Check sheet for the modelled part. Datum: model origin and axes. Units: mm. Face numbers are marked on the shaded views. A direction names the side the tool comes from. Coordinates: 2 decimals unless noted, no trailing zeros. Loops run counter-clockwise (first coordinate to the right, second up) from the corner with the lowest first, then second, coordinate; pieces in that order, holes last. Notation, with made-up numbers: (14.5, 32.25) -> (26.5, 32.25) arc R24 ccw to (26.5, 42.25) -> close; hole circle Ø3 at (-3, -17.5). An arc over 180 degrees is marked (long way). Use CSV: the item, a comma, the result in double quotes.
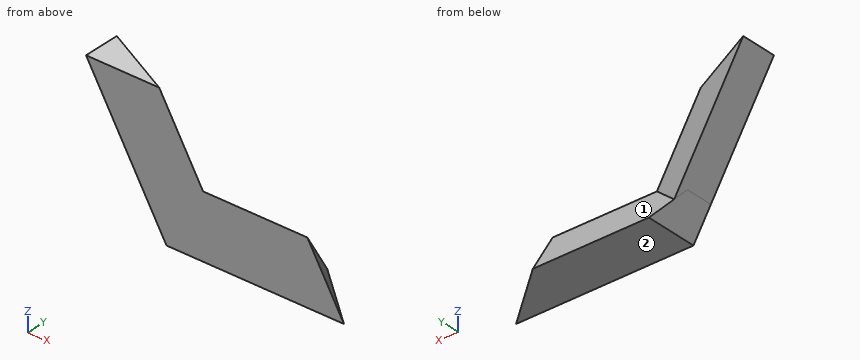
```python
from build123d import *

# Parameters (mm, degrees)
EXTRUDE1_DEPTH          = 153.73
EXTRUDE2_DEPTH          = 127.02
CUT_EXTRUDE1_DEPTH      = 42.954981559
CUT_EXTRUDE2_DEPTH      = 40
CUT_EXTRUDE2_DEPTH_BACK = 60
SKETCH10_W              = 60.093449
SKETCH10_H              = 28.719359
CUT_EXTRUDE3_DEPTH      = 42.954981559


with BuildPart() as part:
    # Sketch1 → Extrude1 (new body)
    with BuildSketch(Plane(origin=(0, 0, 0), x_dir=(0, 0, -1), z_dir=(1, 0, 0))):
        Polygon((0, 0), (0, 41.954981559), (-50, 0), align=None)
    extrude(amount=-EXTRUDE1_DEPTH)

    # Sketch4 → Extrude2 (add)
    with BuildSketch(Plane(origin=(-98.508529611, 0, 170.621778265), x_dir=(0.866025404, 0, 0.5), z_dir=(-0.5, 0, 0.866025404))):
        Polygon((-121.243556529, 28.867513459), (-71.243556529, 0), (-121.243556529, 0), align=None)
    extrude(amount=-EXTRUDE2_DEPTH)

    # Sketch6 → Cut-Extrude1 (cut, through all)
    with BuildSketch(Plane(origin=(0, 0, 0), x_dir=(1, 0, 0), z_dir=(0, 1, 0))):
        Polygon((-161.048753394, -36.457510316), (-140, 0), (-161.048753394, 0), align=None)
    extrude(amount=CUT_EXTRUDE1_DEPTH, mode=Mode.SUBTRACT)

    # Sketch9 → Cut-Extrude2 (cut, two sides)
    with BuildSketch(Plane(origin=(-28.867513459, 0, 50), x_dir=(0.866025404, 0, 0.5), z_dir=(-0.5, 0, 0.866025404))) as cut_extrude2_sk:
        Polygon((33.293903828, 48.675552454), (33.293903828, 0), (0, 0), (-48.675552454, 48.675552454), align=None)
    extrude(amount=CUT_EXTRUDE2_DEPTH, mode=Mode.SUBTRACT)
    extrude(cut_extrude2_sk.sketch, amount=-CUT_EXTRUDE2_DEPTH_BACK, mode=Mode.SUBTRACT)

    # Sketch10 → Cut-Extrude3 (cut, through all)
    with BuildSketch(Plane(origin=(0, 0, 0), x_dir=(1, 0, 0), z_dir=(0, 1, 0))):
        with Locations((-173.7940015, -124.3340965)):
            Rectangle(SKETCH10_W, SKETCH10_H)
    extrude(amount=CUT_EXTRUDE3_DEPTH, mode=Mode.SUBTRACT)


solid = part.part
```
1) Go/stop test with flat-tipped pins: pin 1 Ø6 at (x, y) = (-115, 7.5) entering from -Z; pin 2 Ø8 at (x, y) = (-128, 27.5) entering from +Z; pin 3 Ø4 at (x, y) = (-45, 32.5) entering from +Z; pin 4 Ø1 at (x, z) = (-50.5, 36.5) entering from -Y. Record where each tip stops, or that it passes through.
Answer below:
pin 1,"stops at z = 0"
pin 2,"stops at z = 21.99"
pin 3,"stops at z = 13.65"
pin 4,"stops at y = 0"
2) Thickness scan on line 1 along X through (y, z) = (9, 68.5); line 2 along Z through (x, y) = (-42.5, 34); line 3 along X through (y, z) = (4.5, 25.5). Record the ranges inside material, lowest first. Write a range as from..to.
Answer below:
line 1,"x = -179.55..-139.81"
line 2,"z = 0..5.61"
line 3,"x = -154.72..-19.92"
3) Access from +Z, -Z, +X, -X, +Y, -Y to the whole of each face (thin tool, end or side, straight path). Record for the marked faces 1 and 2.
Answer below:
face 1,"+Z, +X, +Y"
face 2,"-Z, +X, -X, +Y, -Y"
4) Cross-section at C-C on x = -40. Record the boundary of the cut face in (y, z), and give its area (3 significant figures).
Answer below:
outline,"(0, 0) -> (34.64, 0) -> (23.86, 21.57) -> (0, 50) -> close"
area,"970 mm²"
5) Cross-section at B-B on z = 47. Record the boundary of the cut face in (x, y), and give its area (3 significant figures).
Answer below:
outline,"(-167.14, 0) -> (-27.14, 0) -> (-30.04, 2.52) -> (-114.44, 2.52) -> (-167.14, 28.87) -> close"
area,"1,040 mm²"
